The listing builds one solid part. Answer for the finished solid, in the listing's coordinates (mm). Face numbers are marked on the shaded views. A direction names the side the tool comes from. Round coordinates to 2 decimals unless told otherwise and drop trailing zeros. Loops run counter-clockwise (first coordinate to the right, second up) from the corner with the lowest first, then second, coordinate; pieces in that order, holes last. Notation, with made-up numbers: (6.25, 77) -> (24.25, 77) arc R17 cw to (24.25, 82) -> close; hole circle Ø1 at (-2.75, 71.5). An arc over 180 degrees is marked (long way). Use a Markdown table: item, result. Add a question column.
Q1. Section C-C on x = 43 is taken. Give the vertices of the cut face in (y, z).
Q2. Consider line 1 (X direction, y = 62, z = 57); line 2 (Z direction, x = 13.5, y = 22); line 3 (Y direction, x = 20, z = 64.5). Determine where each line is inside the solid, lowest interval first.
Q3. Section A-A on y = 30 is taken. Give the vertices of the cut face in (x, z).
Q4. Given pin 1 Ø3 at (x, z) = (68.5, 72.5) entering from -Y; pin 2 Ø5 at (x, y) = (1, 18) entering from -Z; pin 3 Ø12 at (x, y) = (64, 40) entering from +Z; pin 4 Ø12 at (x, y) = (-55.5, 49) entering from +Z, each flat-ended and moving along its own axis, determine where each tip first touches the part or whether it passes through.
Q5. Which of the six approach directions +Z, -Z, +X, -X, +Y, -Y give full straight-line access (tool end or side, diameter ignored) to the marked faces 1, 2, 3, 4 and 5?
Q6. Section B-B on z = 64.5 is taken. Give the vertices of the cut face in (x, y), then the cut area to 3 significant figures.
Q7. Section D-D on y = 11.5 is taken. Give the vertices of the cut face in (x, z).
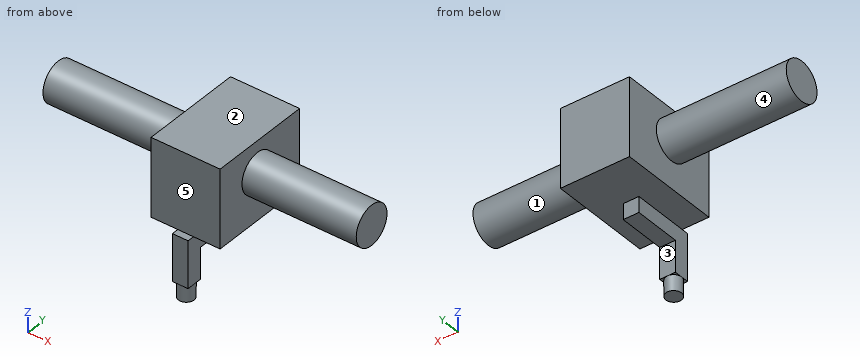
Autodesk Inventor part; units mm, degrees
ref_plane "YZ Plane" through (0, 0, 0) normal (1, 0, 0) x (0, 1, 0)
ref_plane "XZ Plane" through (0, 0, 0) normal (0, 1, 0) x (-1, 0, 0)
ref_plane "XY Plane" through (0, 0, 0) normal (0, 0, 1) x (1, 0, 0)
sketch "Skizze1" plane through (0, 0, 0) normal (0, 0, 1) x (1, 0, 0)
  circle A0 centre (0, 0) radius 5
  dimension "d0" = 10
extrude "Extrusion1" add sketch "Skizze1" along normal blind 10
sketch "Skizze2" plane through (0, 0, 10) normal (0, 0, 1) x (1, 0, 0)
  line L0 (-5, 5) -> (5, 5)
  line L1 (5, 5) -> (5, -5)
  line L2 (5, -5) -> (-5, -5)
  line L3 (-5, -5) -> (-5, 5)
  circle A0 centre (0, 0) radius 5
  dimension "d3" = 10
  dimension "d4" = 10
extrude "Extrusion2" add sketch "Skizze2" along normal blind 30
sketch "Skizze3" plane through (0, 5, 10) normal (0, 1, 0) x (1, 0, 0)
  line L0 (-5, -30) -> (5, -30)
  line L1 (5, -30) -> (-5, -30)
  line L2 (-5, -30) -> (-5, -20)
  line L3 (-5, -20) -> (5, -20)
  line L4 (5, -20) -> (5, -30)
  point P0 (0, 10)
  dimension "d7" = 10
  dimension "d8" = 10
extrude "Extrusion3" add sketch "Skizze3" along normal blind 30
sketch "Skizze5" plane through (0, 0, 40) normal (0, 0, 1) x (1, 0, 0)
  line L0 (-5, -5) -> (-5, 35)
  line L1 (-5, 35) -> (5, 35)
  line L2 (5, 35) -> (5, 25)
  line L3 (5, 25) -> (-5, 25)
  line L4 (-5, 25) -> (-5, 35)
  point P0 (0, 0)
  dimension "d11" = 10
  dimension "d12" = 10
extrude "Extrusion4" add sketch "Skizze5" along normal blind 30
sketch "Skizze6" plane through (-5, 0, 10) normal (-1, 0, 0) x (0, 0, 1)
  line L0 (60, 25) -> (60, 35)
  circle A0 centre (60, 30) radius 12.65
  point P0 (-10, 0)
  dimension "d15" = 25.3
extrude "Extrusion5" add sketch "Skizze6" along normal mid plane 200
sketch "Skizze7" plane through (0, 0, 40) normal (0, 0, 1) x (1, 0, 0)
  line L0 (-22.05, -0.6125) -> (22.05, -0.6125)
  line L1 (22.05, -0.6125) -> (22.05, 64.7208)
  line L2 (22.05, 64.7208) -> (-22.05, 64.7208)
  line L3 (-22.05, 64.7208) -> (-22.05, -0.6125)
  line L4 (-5, 5) -> (-5, 35)
  point P0 (0, 0)
  dimension "d18" = 44.1
  dimension "d19" = 17.05
extrude "Extrusion6" add sketch "Skizze7" along normal blind 50
properties part number "ONLY_Inventor_inv1"
Checked values:
| question | item | result |
|---|---|---|
| 1 | outline | circle Ø25.3 at (30, 70) |
| 2 | line 1 | x = -22.05 to 22.05 |
| 2 | line 2 | z = 40 to 90 |
| 2 | line 3 | y = -0.61 to 64.72 |
| 3 | outline | (-105, 57.35) -> (-22.05, 57.35) -> (-22.05, 40) -> (-5, 40) -> (-5, 30) -> (5, 30) -> (5, 40) -> (22.05, 40) -> (22.05, 57.35) -> (95, 57.35) -> (95, 82.65) -> (22.05, 82.65) -> (22.05, 90) -> (-22.05, 90) -> (-22.05, 82.65) -> (-105, 82.65) -> close |
| 4 | pin 1 | stops at y = 17.39 |
| 4 | pin 2 | stops at z = 30 |
| 4 | pin 3 | stops at z = 82 |
| 4 | pin 4 | passes through |
| 5 | face 1 | +X |
| 5 | face 2 | +Z, +X, -X, +Y, -Y |
| 5 | face 3 | -Z, +X, -X, +Y |
| 5 | face 4 | -X |
| 5 | face 5 | +Z, +X, -X, -Y |
| 6 | outline | (-105, 18.61) -> (-22.05, 18.61) -> (-22.05, -0.61) -> (22.05, -0.61) -> (22.05, 18.61) -> (95, 18.61) -> (95, 41.39) -> (22.05, 41.39) -> (22.05, 64.72) -> (-22.05, 64.72) -> (-22.05, 41.39) -> (-105, 41.39) -> close |
| 6 | area | 6,430 mm2 |
| 7 | outline | (-22.05, 40) -> (-5, 40) -> (-5, 30) -> (5, 30) -> (5, 40) -> (22.05, 40) -> (22.05, 90) -> (-22.05, 90) -> close |
